```python
from build123d import *

# Parameters (mm, degrees)
F0_W           = 250
F0_H           = 200
F1_DEPTH       = 10
F3_D           = 6
F3_CSINK_D     = 12
F3_CSINK_ANGLE = 90
F4_W           = 50
F4_H           = 10
F5_DEPTH       = 10


with BuildPart() as f1:
    # F0 (on Top) → F1 (new body)
    with BuildSketch(Plane.XY):
        Rectangle(F0_W, F0_H)
    extrude(amount=F1_DEPTH)

    # F3 (through all)
    with Locations(Plane.XY.offset(10)):
        with Locations((-98.94, 81.645), (98.94, 81.645), (98.94, -81.645), (-98.94, -81.645)):
            CounterSinkHole(F3_D / 2, F3_CSINK_D / 2, counter_sink_angle=F3_CSINK_ANGLE)

    # F4 (on Top) → F5 (join)
    with BuildSketch(Plane.XY):
        Rectangle(F4_W, F4_H)
    extrude(amount=-F5_DEPTH)


solid = f1.part
```
Model file for the job. Use its own axes, mm. A direction names the side the tool comes from. Coordinates: 2 decimals unless noted, no trailing zeros. Loops run counter-clockwise (first coordinate to the right, second up) from the corner with the lowest first, then second, coordinate; pieces in that order, holes last. Notation, with made-up numbers: (0, 30.5) - (28, 30.5) arc R29 cw to (28, 63.5) - close; hole circle Ø9 at (-39.5, 4.5). An arc over 180 degrees is marked (long way). Answer as a JSON object with one key per item and string values. Group by question number.
(1) Flat gauge pins, fed straight in: pin 1 (5 mm diameter, centred on y = -1.5, z = -4, fed in from +X); pin 2 (9.5 mm diameter, centred on x = 98.94, y = -81.645, fed in from +Z); pin 3 (11 mm diameter, centred on x = -12, z = -5, fed in from +Y); pin 4 (5 mm diameter, centred on x = 58.5, y = 23.5, fed in from -Z). Where does each tip first touch, or does it go through?
(2) Cut at C-C (y = -54). Give the cut face in (x, z), then the cut area to 3 significant figures.
(3) Two-plate mould, pull along X, no slides. Class faces 1 (the face through (-100.39, 78.85, 7.15)), 2 (the face through (25, 0, -5)), 3 (the face through (-25, 0, -5)): released by +X, released by -X, zero draft, split by the parting line, or undercut.
(4) Cut at A-A (x = -98.94). Give the cut face in (y, z) (3 decimals).
(5) Tool access for faces 4 (the face through (97.49, 78.85, 7.15)), 5 (the face through (0, 5, -5)), 6 (the face through (0, -5, -5)): list every direction of +Z, -Z, +X, -X, +Y, -Y with a clear straight run to the whole face (end or side of a thin tool).
(6) Cut at D-D (z = -5.75). Give the cut face in (x, y), then the cut area to 3 significant figures.
(7) Probe line 1 along Y through (x, z) = (98.94, 5.75) (3 decimals); line 2 along X through (y, z) = (-81, 8.25); line 3 along Z through (x, y) = (99, -20). List the from-to ranges inside material, lowest first.
(8) Cut at B-B (x = -15). Give the cut face in (y, z).
Geometry says:
{
 "1": {"pin 1": "stops at x = 25", "pin 2": "stops at z = 8.75", "pin 3": "stops at y = 100", "pin 4": "stops at z = 0"},
 "2": {"outline": "(-125, 0) - (125, 0) - (125, 10) - (-125, 10) - close", "area": "2,500 mm^2"},
 "3": {"face 1": "undercut", "face 2": "released by +X", "face 3": "released by -X"},
 "4": {"outline": "(-100, 0) - (-84.645, 0) - (-84.645, 7) - (-87.645, 10) - (-100, 10) - close; (-78.645, 0) - (78.645, 0) - (78.645, 7) - (75.645, 10) - (-75.645, 10) - (-78.645, 7) - close; (84.645, 0) - (100, 0) - (100, 10) - (87.645, 10) - (84.645, 7) - close"},
 "5": {"face 4": "+Z", "face 5": "-Z, +X, -X, +Y", "face 6": "-Z, +X, -X, -Y"},
 "6": {"outline": "(-25, -5) - (25, -5) - (25, 5) - (-25, 5) - close", "area": "500 mm^2"},
 "7": {"line 1": "y = -100 to -84.645, -78.645 to 78.645, 84.645 to 100", "line 2": "x = -125 to -103.14, -94.74 to 94.74, 103.14 to 125", "line 3": "z = 0 to 10"},
 "8": {"outline": "(-100, 0) - (-5, 0) - (-5, -10) - (5, -10) - (5, 0) - (100, 0) - (100, 10) - (-100, 10) - close"}
}
